Read the model definition and answer for the solid it produces. Units are mm, in the model's axes. A direction names the side the tool comes from. Round coordinates to 2 decimals unless told otherwise and drop trailing zeros. Write each loop counter-clockwise with the first axis right and the second up, starting at its lowest first coordinate (ties: lowest second). Pieces come first, ordered by that corner, then holes. Notation, with made-up numbers: (65.5, 6) - (90.5, 6) arc R26 ccw to (90.5, 25) - close; hole circle Ø6 at (50.25, 65). An arc over 180 degrees is marked (long way). Use one line per item in the form item = value. Start each with the question number.
1) The part is cut by section C-C, the plane z = -19.5. Give the vertices of the cut face in (x, y), plus the area to 3 significant figures.
2) The part is cut by section D-D, the plane z = -8.5. Give the vertices of the cut face in (x, y), plus the area to 3 significant figures.
3) Consider line 1 along Z through (x, y) = (1, 10); line 2 along X through (y, z) = (13.5, -16.5). Determine where each line is inside the solid, lowest interval first. Write a range as from..to.
4) The part is cut by section A-A, the plane y = 12. Give the vertices of the cut face in (x, z), plus the area to 3 significant figures.
5) The part is cut by section B-B, the plane x = 4. Give the vertices of the cut face in (y, z), plus the area to 3 significant figures.
6) For a pull along Z with two mould halves and no side action, classify faces 4 (the face through (0.66, 0.63, -12.17)), 5 (the face through (5, 1, 0)), 6 (the face through (2.553, 0.592, -4.445)) as released by +Z, released by -Z, zero draft, split by the parting line, or undercut.
7) For faces 1 (the face through (17.88, 1, -12)), 2 (the face through (1.2, 10, -12)), 3 (the face through (9, 1, -7)), determine the directions among +Z, -Z, +X, -X, +Y, -Y from which every point of the face is accessible in a straight line to the end or side of a thin tool.
8) Each of these flat-tipped pins is pushed along its axis until it touches: pin 1 (4.5 mm diameter, centred on y = 12, z = -16, fed in from +X); pin 2 (10 mm diameter, centred on x = 9.5, z = -3.5, fed in from +Y). Where does it stop, or does it pass through?
from build123d import *

# Parameters (mm, degrees)
SKETCH1_W           = 24
SKETCH1_H           = 17
SKETCH1_R           = 2.5
BOSS_EXTRUDE1_DEPTH = 1.2
SKETCH3_W           = 17.88
SKETCH3_H           = 24
BOSS_EXTRUDE3_DEPTH = 1.2
FILLET1_R           = 1
FILLET2_R           = 2.2


with BuildPart() as part:
    # Sketch1 → Boss-Extrude1 (new body)
    with BuildSketch(Plane(origin=(0, 0, 0), x_dir=(0, 0, -1), z_dir=(1, 0, 0))):
        with Locations((12, 8.5)):
            Rectangle(SKETCH1_W, SKETCH1_H)
        with Locations((4.5, 12)):
            Circle(SKETCH1_R, mode=Mode.SUBTRACT)
        with Locations((19.5, 12)):
            Circle(SKETCH1_R, mode=Mode.SUBTRACT)
    extrude(amount=BOSS_EXTRUDE1_DEPTH)

    # Sketch3 → Boss-Extrude3 (add)
    with BuildSketch(Plane(origin=(0, 0, 0), x_dir=(1, 0, 0), z_dir=(0, 1, 0))):
        with Locations((8.94, 12)):
            Rectangle(SKETCH3_W, SKETCH3_H)
        with BuildLine():
            Line((5.052758316, 22), (12.947241684, 22))
            ThreePointArc((12.947241684, 22), (15.447241684, 19.5), (12.947241684, 17))
            Line((12.947241684, 17), (5.052758316, 17))
            ThreePointArc((5.052758316, 17), (2.552758316, 19.5), (5.052758316, 22))
        make_face(mode=Mode.SUBTRACT)
        with BuildLine():
            Line((5.052758316, 7), (12.947241684, 7))
            ThreePointArc((12.947241684, 7), (15.447241684, 4.5), (12.947241684, 2))
            Line((12.947241684, 2), (5.052758316, 2))
            ThreePointArc((5.052758316, 2), (2.552758316, 4.5), (5.052758316, 7))
        make_face(mode=Mode.SUBTRACT)
    extrude(amount=BOSS_EXTRUDE3_DEPTH)

    # Fillet1
    fillet1_edges = [part.edges().sort_by_distance(p)[0] for p in [
        (1.2, 1.2, -12),
    ]]
    fillet(fillet1_edges, radius=FILLET1_R)

    # Fillet2
    fillet2_edges = [part.edges().sort_by_distance(p)[0] for p in [
        (0, 0, -12),
    ]]
    fillet(fillet2_edges, radius=FILLET2_R)


solid = part.part
Geometry results:
q1.outline = (0, 2.2) arc R2.2 ccw to (2.2, 0) - (2.55, 0) - (2.55, 1.2) - (2.2, 1.2) arc R1 cw to (1.2, 2.2) - (1.2, 9.5) - (0, 9.5) - close; (0, 14.5) - (1.2, 14.5) - (1.2, 17) - (0, 17) - close; (15.45, 0) - (17.88, 0) - (17.88, 1.2) - (15.45, 1.2) - close
q1.area = 18.1 mm2
q2.outline = (0, 2.2) arc R2.2 ccw to (2.2, 0) - (17.88, 0) - (17.88, 1.2) - (2.2, 1.2) arc R1 cw to (1.2, 2.2) - (1.2, 17) - (0, 17) - close
q2.area = 39.6 mm2
q3.line_1 = -24..-21, -18..-6, -3..0
q3.line_2 = 0..1.2
q4.outline = (0, -24) - (1.2, -24) - (1.2, -22) - (0, -22) - close; (0, -17) - (1.2, -17) - (1.2, -7) - (0, -7) - close; (0, -2) - (1.2, -2) - (1.2, 0) - (0, 0) - close
q4.area = 16.8 mm2
q5.outline = (0, -24) - (1.2, -24) - (1.2, -21.77) - (0, -21.77) - close; (0, -17.23) - (1.2, -17.23) - (1.2, -6.77) - (0, -6.77) - close; (0, -2.23) - (1.2, -2.23) - (1.2, 0) - (0, 0) - close
q5.area = 17.9 mm2
q6.face_4 = zero draft
q6.face_5 = released by +Z
q6.face_6 = undercut
q7.face_1 = +Z, -Z, +X, +Y, -Y
q7.face_2 = +Z, -Z, +X, +Y
q7.face_3 = +Y, -Y
q8.pin_1 = 1.2
q8.pin_2 = 1.2
